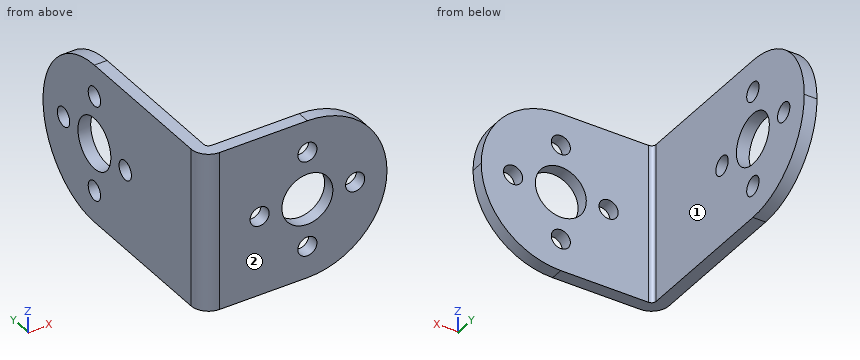
```python
from build123d import *

# Parameters (mm, degrees)
SKETCH1_R                    = 1.5
SKETCH1_R_2                  = 4
BASE_FLANGE1_DEPTH           = 2
SKETCHED_START               = -32.5
SKETCHED_BEND1_OUTLINE_W     = 2
SKETCHED_BEND1_OUTLINE_H     = 25
SKETCHED_BEND1_DEPTH         = 36
SKETCHED_START_2             = 3.766161716
SKETCHED_BEND1_2_OUTLINE_R   = 1.5
SKETCHED_BEND1_2_OUTLINE_R_2 = 4
SKETCHED_BEND1_2_DEPTH       = 1.733838284
SKETCHED_START_3             = 3.5
SKETCHED_BEND1_3_OUTLINE_R   = 1.5
SKETCHED_BEND1_3_OUTLINE_R_2 = 4
SKETCHED_BEND1_3_DEPTH       = 2.7366
SKETCHED_START_4             = -12.5
SKETCHED_BEND1_4_DEPTH       = 25


with BuildPart() as part:
    # Base-Flange1: sheet metal written as solids
    # Sketch1 → Base-Flange1 (new body)
    with BuildSketch(Plane(origin=(0, 0, 0), x_dir=(1, 0, 0), z_dir=(0, 1, 0))):
        with BuildLine():
            Line((-32.5, -0.001), (-32.5, 0.001))
            ThreePointArc((-32.5, 0.001), (-28.839127658, 8.839127658), (-20.001, 12.5))
            Line((-20.001, 12.5), (20.001, 12.5))
            ThreePointArc((20.001, 12.5), (28.839127658, 8.839127658), (32.5, 0.001))
            Line((32.5, 0.001), (32.5, -0.001))
            ThreePointArc((32.5, -0.001), (28.839127658, -8.839127658), (20.001, -12.5))
            Line((20.001, -12.5), (-20.001, -12.5))
            ThreePointArc((-20.001, -12.5), (-28.839127658, -8.839127658), (-32.5, -0.001))
        make_face()
        with Locations(Location((12.501, 0.000250009, 0), (0, 0, 270))):
            Circle(SKETCH1_R, mode=Mode.SUBTRACT)
        with Locations(Location((20.001, 0.000250009, 0), (0, 0, 270))):
            Circle(SKETCH1_R_2, mode=Mode.SUBTRACT)
        with Locations(Location((20.001, -7.499749991, 0), (0, 0, 270))):
            Circle(SKETCH1_R, mode=Mode.SUBTRACT)
        with Locations(Location((27.501, 0.000250009, 0), (0, 0, 270))):
            Circle(SKETCH1_R, mode=Mode.SUBTRACT)
        with Locations(Location((20.001, 7.500250009, 0), (0, 0, 270))):
            Circle(SKETCH1_R, mode=Mode.SUBTRACT)
        with Locations(Location((-20.001, 7.499, 0), (0, 0, 270))):
            Circle(SKETCH1_R, mode=Mode.SUBTRACT)
        with Locations(Location((-27.500999963, -0.000250009, 0), (0, 0, 270))):
            Circle(SKETCH1_R, mode=Mode.SUBTRACT)
        with Locations(Location((-12.501000067, 0, 0), (0, 0, 270))):
            Circle(SKETCH1_R, mode=Mode.SUBTRACT)
        with Locations(Location((-20.001, -7.501, 0), (0, 0, 270))):
            Circle(SKETCH1_R, mode=Mode.SUBTRACT)
        with Locations(Location((-20.001, -0.001, 0), (0, 0, 270))):
            Circle(SKETCH1_R_2, mode=Mode.SUBTRACT)
    extrude(amount=-BASE_FLANGE1_DEPTH)

    # Sketched Bend1: read off the stored shape, not the designer's step
    # Sketched Bend1 outline → Sketched Bend1 (cut)
    with BuildSketch(Plane.YZ.offset(SKETCHED_START)):
        with Locations((-1, 0)):
            Rectangle(SKETCHED_BEND1_OUTLINE_W, SKETCHED_BEND1_OUTLINE_H)
    extrude(amount=SKETCHED_BEND1_DEPTH, mode=Mode.SUBTRACT)

    # Sketched Bend1 2 outline → Sketched Bend1 2 (add)
    with BuildSketch(Plane.YZ.offset(SKETCHED_START_2)):
        with BuildLine():
            ThreePointArc((36.745355099, 0.001), (33.084482757, 8.839127658), (24.246355099, 12.5))
            Line((24.246355099, 12.5), (0, 12.5))
            Line((0, 12.5), (0, -12.5))
            Line((0, -12.5), (24.246355099, -12.5))
            ThreePointArc((24.246355099, -12.5), (33.084482757, -8.839127658), (36.745355099, -0.001))
            Line((36.745355099, -0.001), (36.745355099, 0.001))
        make_face()
        with Locations((24.246355099, -7.499)):
            Circle(SKETCHED_BEND1_2_OUTLINE_R, mode=Mode.SUBTRACT)
        with Locations((16.746355166, 0)):
            Circle(SKETCHED_BEND1_2_OUTLINE_R, mode=Mode.SUBTRACT)
        with Locations((24.246355099, 0.001)):
            Circle(SKETCHED_BEND1_2_OUTLINE_R_2, mode=Mode.SUBTRACT)
        with Locations((31.746355061, 0.000250009)):
            Circle(SKETCHED_BEND1_2_OUTLINE_R, mode=Mode.SUBTRACT)
        with Locations((24.246355099, 7.501)):
            Circle(SKETCHED_BEND1_2_OUTLINE_R, mode=Mode.SUBTRACT)
    extrude(amount=SKETCHED_BEND1_2_DEPTH)

    # Sketched Bend1 3 outline → Sketched Bend1 3 (add)
    with BuildSketch(Plane.YZ.offset(SKETCHED_START_3)):
        with BuildLine():
            ThreePointArc((36.745355099, 0.001), (33.084482757, 8.839127658), (24.246355099, 12.5))
            Line((24.246355099, 12.5), (0, 12.5))
            Line((0, 12.5), (0, -12.5))
            Line((0, -12.5), (24.246355099, -12.5))
            ThreePointArc((24.246355099, -12.5), (33.084482757, -8.839127658), (36.745355099, -0.001))
            Line((36.745355099, -0.001), (36.745355099, 0.001))
        make_face()
        with Locations((24.246355099, -7.499)):
            Circle(SKETCHED_BEND1_3_OUTLINE_R, mode=Mode.SUBTRACT)
        with Locations((16.746355166, 0)):
            Circle(SKETCHED_BEND1_3_OUTLINE_R, mode=Mode.SUBTRACT)
        with Locations((24.246355099, 0.001)):
            Circle(SKETCHED_BEND1_3_OUTLINE_R_2, mode=Mode.SUBTRACT)
        with Locations((31.746355061, 0.000250009)):
            Circle(SKETCHED_BEND1_3_OUTLINE_R, mode=Mode.SUBTRACT)
        with Locations((24.246355099, 7.501)):
            Circle(SKETCHED_BEND1_3_OUTLINE_R, mode=Mode.SUBTRACT)
    extrude(amount=SKETCHED_BEND1_3_DEPTH)

    # Sketched Bend1 4 outline → Sketched Bend1 4 (cut)
    with BuildSketch(Plane.XY.offset(SKETCHED_START_4)):
        with BuildLine():
            ThreePointArc((6.2366, -2), (4.301531583, -1.198468417), (3.5, 0.7366))
            Line((3.5, 0.7366), (3.5, -2))
            Line((3.5, -2), (6.2366, -2))
        make_face()
        with BuildLine():
            Line((5.5, 36.745355099), (5.5, 0.7366))
            ThreePointArc((5.5, 0.7366), (5.715745145, 0.215745145), (6.2366, 0))
            Line((6.2366, 0), (6.2366, 36.745355099))
            Line((6.2366, 36.745355099), (5.5, 36.745355099))
        make_face()
    extrude(amount=SKETCHED_BEND1_4_DEPTH, mode=Mode.SUBTRACT)


solid = part.part
```
Work out the finished part from the listing and answer in its coordinate system (mm). Face numbers are marked on the shaded views. A direction names the side the tool comes from. Coordinates: 2 decimals unless noted, no trailing zeros. Order: outer loops, then holes, each group sorted by start corner. A loop starts at its lowest first (then second) coordinate and runs counter-clockwise, first axis right, second up. Notation, with made-up numbers: M 23,16 L 55,16 A25 ccw 55,41 Z; hole C 51.5,80 d8. An arc over 180 degrees is marked long. Use CSV: the item, a comma, the result in double quotes.
1) Section D-D on x = 13.25 is taken. Write down the section's boundary in (y, z), plus the area to 3 significant figures.
Worked out:
outline,"M -2,-12.5 L 0,-12.5 L 0,-1.3 L -2,-1.3 Z; M -2,1.3 L 0,1.3 L 0,12.5 L -2,12.5 Z"
area,"44.8 mm^2"
2) Section A-A on x = 22 is taken. Write down the section's boundary in (y, z).
Worked out:
outline,"M -2,-12.34 L 0,-12.34 L 0,-3.46 L -2,-3.46 Z; M -2,3.46 L 0,3.46 L 0,12.34 L -2,12.34 Z"
3) Section C-C on y = 19 is taken. Write down the section's boundary in (x, z).
Worked out:
outline,"M 3.5,-12.5 L 5.5,-12.5 L 5.5,12.5 L 3.5,12.5 Z"
4) For the marked faces 1 and 2, determine the directions among +Z, -Z, +X, -X, +Y, -Y from which every point of the face is accessible in a straight line to the end or side of a thin tool.
Worked out:
face 1,"+Z, -Z, +X, +Y"
face 2,"+Z, -Z, +X, -X, -Y"
5) Consider line 1 (X direction, y = 20, z = 3.25); line 2 (Y direction, x = 14, z = -6). Determine where each line is inside the solid, lowest interval first. Write a range as [from, to].
Worked out:
line 1,"x = [3.5, 5.5]"
line 2,"y = [-2, 0]"
6) Section B-B on z = 0.75 is taken. Count the separate pieces of the cut face and the enclosed holes in it, plus the area to 3 significant figures.
Worked out:
separate pieces,"7"
enclosed holes,"0"
area,"77.7 mm^2"
7) Flat-ended cylindrical pins translate along their axes: pin 1 Ø2 at (y, z) = (8, -5.5) entering from +X; pin 2 Ø6 at (x, z) = (13.5, 7.5) entering from +Y; pin 3 Ø1.8 at (y, z) = (24.25, 7.5) entering from -X. Find the tip coordinate at first contact, or state that the pin passes through.
Worked out:
pin 1,"stops at x = 5.5"
pin 2,"stops at y = 0"
pin 3,"passes through"
